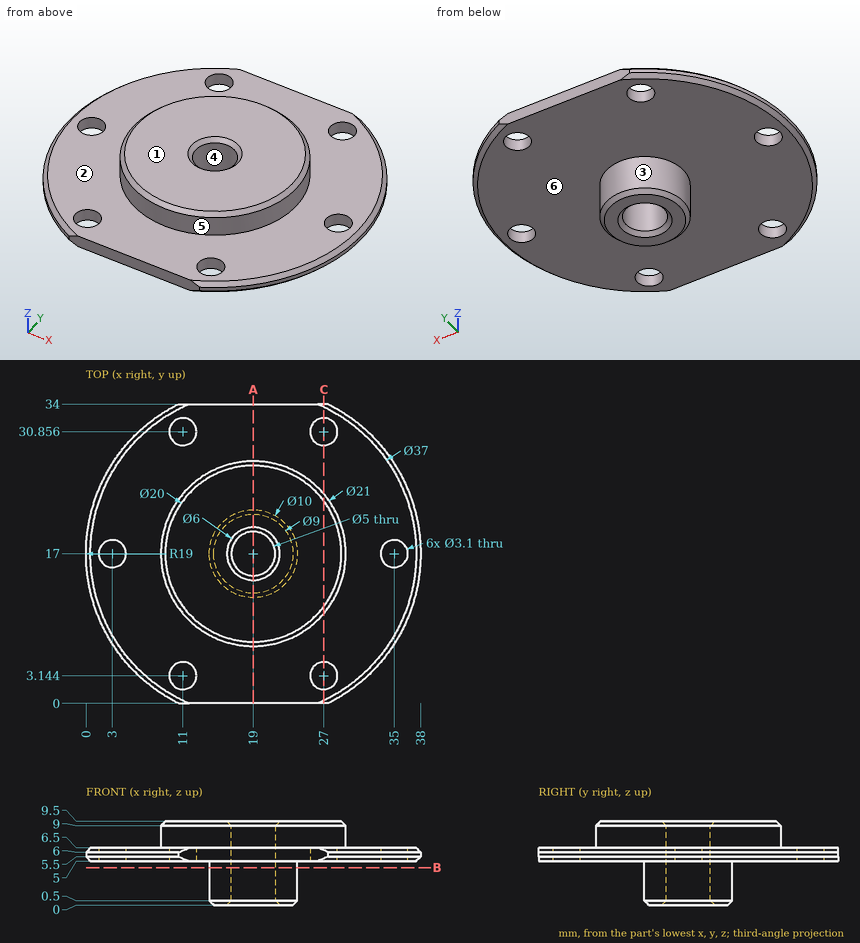
Study the drawing (mm; zero at the part's minimum x, y, z) and answer. A direction names the side the tool comes from. Coordinates: 2 decimals unless noted, no trailing zeros. Write each loop counter-clockwise with the first axis right and the second up, starting at its lowest first coordinate (ties: lowest second). Pieces come first, ordered by that corner, then holes. Notation, with made-up numbers: (47, 82.25) - (100, 82.25) arc R28 cw to (100, 111.25) - close; hole circle Ø11 at (-38, 13). An arc over 180 degrees is marked (long way). Answer as a JSON object with one key per item and string values.
Q1. Which of the six approach directions +Z, -Z, +X, -X, +Y, -Y give full straight-line access (tool end or side, diameter ignored) to the marked faces 1, 2 and 3?
Results list:
{"face 1": "+Z, +X, -X, +Y, -Y", "face 2": "+Z", "face 3": "-Z"}
Q2. Given pin 1 Ø5 at (x, y) = (11, 30.86) entering from +Z; pin 2 Ø5 at (x, z) = (4.5, 5) entering from +Y; pin 3 Ø4 at (x, y) = (11, 3.14) entering from -Z, each flat-ended and moving along its own axis, determine where each tip first touches the part or whether it passes through.
Results list:
{"pin 1": "stops at z = 6.5", "pin 2": "stops at y = 31.69", "pin 3": "stops at z = 5"}
Q3. Find section A-A (x = 19). Write down the section's boundary in (y, z).
Results list:
{"outline": "(0, 5) - (12, 5) - (12, 0.5) - (12.5, 0) - (14, 0) - (14.5, 0.5) - (14.5, 9) - (14, 9.5) - (7, 9.5) - (6.5, 9) - (6.5, 6.5) - (0, 6.5) - close; (19.5, 0.5) - (20, 0) - (21.5, 0) - (22, 0.5) - (22, 5) - (34, 5) - (34, 6.5) - (27.5, 6.5) - (27.5, 9) - (27, 9.5) - (20, 9.5) - (19.5, 9) - close"}
Q4. Consider L1, parallel to Y at x = 27, z = 5.5; L2, parallel to Z at x = 34.5, y = 27; L3, parallel to X at y = 15, z = 7.5 (1 decimal). Determine where each line is inside the solid, lowest interval first. Write a range as from..to.
Results list:
{"L1": "y = 0..1.59, 4.69..29.31, 32.41..34", "L2": "z = 5..6.5", "L3": "x = 8.7..17.5, 20.5..29.3"}
Q5. Find section B-B (z = 4.25). Write down the section's boundary in (x, y).
Results list:
{"outline": "circle Ø10 at (19, 17); hole circle Ø5 at (19, 17)"}
Q6. Find section C-C (x = 27). State how many separate pieces and enclosed holes the cut face has.
Results list:
{"separate pieces": "3", "enclosed holes": "0"}
Q7. For a pull along Y with two mould halves and no side action, classify the marked faces 4, 5 and 6 as pulls with the +Y half, pulls with the -Y half, needs draft (parallel to the pull), parting line crosses it, or undercut.
Results list:
{"face 4": "undercut", "face 5": "parting line crosses it", "face 6": "needs draft"}
